CAD build for the part. Positions are in the model's coordinates, mm. Face numbers are marked on the shaded views. A direction names the side the tool comes from. Give positions to 0.01 mm unless a question says otherwise; leave off trailing zeros. Write each loop counter-clockwise with the first axis right and the second up, starting at its lowest first coordinate (ties: lowest second). Pieces come first, ordered by that corner, then holes. Notation, with made-up numbers: (38, 42) - (77, 42) arc R23 ccw to (77, 66) - close; hole circle Ø7 at (67.25, -15). An arc over 180 degrees is marked (long way). Put each result on its own line as item: value. Start each with the question number.
1. Wall check: line 1 (Z direction, x = 21, y = -6); line 2 (Z direction, x = -10.5, y = 23.5); line 3 (X direction, y = 0, z = -5). Give the ranges that are in metal, low to high.
2. Tool access for the marked faces 1, 2 and 3: list every direction of +Z, -Z, +X, -X, +Y, -Y with a clear straight run to the whole face (end or side of a thin tool).
3. Cut at B-B on z = 5.5. List the corners of the cut face in (x, y).
4. Drop flat-ended pins along their axis: pin 1 (1 mm diameter, centred on x = -17, y = 15, fed in from -Z); pin 2 (8 mm diameter, centred on x = -7.5, z = 12, fed in from +Y); pin 3 (5 mm diameter, centred on y = -9.5, z = 9, fed in from -X) (3 decimals). Give the stop position or say it passes through.
5. Cut at A-A on x = 0. List the corners of the cut face in (y, z).
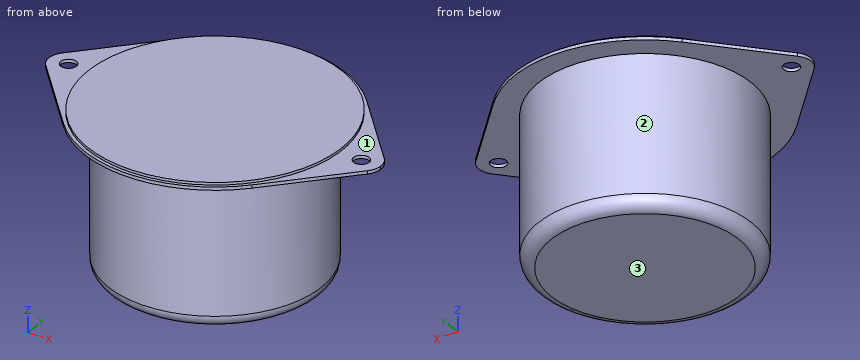
from build123d import *

# Parameters (mm, degrees)
F2_R     = 1.5875
F3_DEPTH = 0.635
F4_R     = 2.54


with BuildPart() as f1:
    # F0 (on Front) → F1 (revolve)
    with BuildSketch(Plane.XZ):
        Polygon((26.0985, 14.351), (26.0985, 14.986), (25.4, 14.986), (25.4, 15.494), (0, 15.494), (0, -15.494), (21.336, -15.494), (21.336, 14.351), align=None)
    revolve(axis=Axis((0, 0, -4.175231), (0, 0, -1)))

    # F2 (on face) → F3 (join, through all)
    with BuildSketch(Plane.XY.offset(14.986)):
        with BuildLine():
            ThreePointArc((19.326104, -17.539481), (24.346602, -9.400781), (26.0985, 0))
            ThreePointArc((26.0985, 0), (24.346602, 9.400781), (19.326104, 17.539481))
            ThreePointArc((19.326104, 17.539481), (0, 26.0985), (-19.326104, 17.539481))
            ThreePointArc((-19.326104, 17.539481), (-26.0985, 0), (-19.326104, -17.539481))
            ThreePointArc((-19.326104, -17.539481), (0, -26.0985), (19.326104, -17.539481))
        make_face()
        with BuildLine():
            ThreePointArc((19.326104, 17.539481), (24.346602, 9.400781), (26.0985, 0))
            ThreePointArc((26.0985, 0), (24.346602, -9.400781), (19.326104, -17.539481))
            Line((19.326104, -17.539481), (32.920329, -2.560508))
            ThreePointArc((32.920329, -2.560508), (26.289, 0), (32.920329, 2.560508))
            Line((32.920329, 2.560508), (19.326104, 17.539481))
        make_face()
        with BuildLine():
            ThreePointArc((-19.326104, -17.539481), (-26.0985, 0), (-19.326104, 17.539481))
            Line((-19.326104, 17.539481), (-32.920329, 2.560508))
            ThreePointArc((-32.920329, 2.560508), (-28.726623, 3.554248), (-26.289, 0))
            ThreePointArc((-26.289, 0), (-28.726623, -3.554248), (-32.920329, -2.560508))
            Line((-32.920329, -2.560508), (-19.326104, -17.539481))
        make_face()
        with BuildLine():
            ThreePointArc((33.909, 0), (33.653248, 1.372377), (32.920329, 2.560508))
            ThreePointArc((32.920329, 2.560508), (26.289, 0), (32.920329, -2.560508))
            ThreePointArc((32.920329, -2.560508), (33.653248, -1.372377), (33.909, 0))
        make_face()
        with Locations((29.972, 0)):
            Circle(F2_R, mode=Mode.SUBTRACT)
        with BuildLine():
            ThreePointArc((-26.289, 0), (-28.726623, 3.554248), (-32.920329, 2.560508))
            ThreePointArc((-32.920329, 2.560508), (-33.909, 0), (-32.920329, -2.560508))
            ThreePointArc((-32.920329, -2.560508), (-28.726623, -3.554248), (-26.289, 0))
        make_face()
        with Locations((-29.972, 0)):
            Circle(F2_R, mode=Mode.SUBTRACT)
    extrude(amount=-F3_DEPTH)

    # F4
    f4_edges = [f1.edges().sort_by_distance(p)[0] for p in [
        (-21.336, 0, -15.494),
    ]]
    fillet(f4_edges, radius=F4_R)


solid = f1.part
Report:
1. line 1: z = 14.35 to 15.49
1. line 2: z = 14.35 to 14.99
1. line 3: x = -21.34 to 21.34
2. face 1: +Z
2. face 2: -Z
2. face 3: -Z, +X, -X, +Y, -Y
3. outline: circle Ø42.67 at (0, 0)
4. pin 1: stops at z = 14.35
4. pin 2: stops at y = 25.75
4. pin 3: stops at x = -20.155
5. outline: (-26.1, 14.35) - (-21.34, 14.35) - (-21.34, -12.95) arc R2.54 ccw to (-18.8, -15.49) - (18.8, -15.49) arc R2.54 ccw to (21.34, -12.95) - (21.34, 14.35) - (26.1, 14.35) - (26.1, 14.99) - (25.4, 14.99) - (25.4, 15.49) - (-25.4, 15.49) - (-25.4, 14.99) - (-26.1, 14.99) - close
